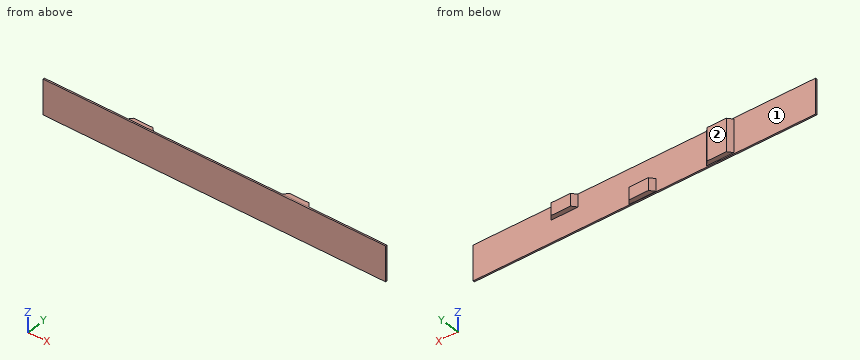
from build123d import *

# Parameters (mm, degrees)
SKETCH1_W           = 2200
SKETCH1_H           = 225
BOSS_EXTRUDE1_DEPTH = 10
BOSS_EXTRUDE2_START = 30
BOSS_EXTRUDE2_DEPTH = 80
BOSS_EXTRUDE3_START = -30
BOSS_EXTRUDE3_DEPTH = 80
BOSS_EXTRUDE4_DEPTH = 105


with BuildPart() as part:
    # Sketch1 → Boss-Extrude1 (new body)
    with BuildSketch(Plane(origin=(0, 0, 0), x_dir=(1, 0, 0), z_dir=(0, 1, 0))):
        Rectangle(SKETCH1_W, SKETCH1_H)
    extrude(amount=BOSS_EXTRUDE1_DEPTH)

    # Sketch2 → Boss-Extrude2 (add)
    with BuildSketch(Plane.XY.offset(BOSS_EXTRUDE2_START)):
        Polygon((425, 10), (450, 40), (575, 40), (600, 10), align=None)
    extrude(amount=BOSS_EXTRUDE2_DEPTH)

    # Sketch3 → Boss-Extrude3 (add)
    with BuildSketch(Plane.XY.offset(BOSS_EXTRUDE3_START)):
        Polygon((75, 40), (-50, 40), (-75, 10), (100, 10), align=None)
    extrude(amount=-BOSS_EXTRUDE3_DEPTH)

    # Sketch4 → Boss-Extrude4 (add, symmetric)
    with BuildSketch(Plane.XY):
        Polygon((-425, 40), (-550, 40), (-575, 10), (-400, 10), align=None)
    extrude(amount=BOSS_EXTRUDE4_DEPTH, both=True)


solid = part.part
The model under review builds one solid part; all positions refer to its coordinate system, in mm. Face numbers are marked on the shaded views. Coordinates: 2 decimals unless noted, no trailing zeros. Loops run counter-clockwise (first coordinate to the right, second up) from the corner with the lowest first, then second, coordinate; pieces in that order, holes last. Notation, with made-up numbers: (31.25, 26.25) -> (80.25, 26.25) arc R25 cw to (80.25, 63.25) -> close; hole circle Ø1 at (30, -17). An arc over 180 degrees is marked (long way). Use a Markdown table: item, result. Add a question column.
1. Clearance check with flat-ended pins moving along their axes: pin 1 Ø15 at (x, y) = (-20, 23.5) entering from +Z; pin 2 Ø1 at (y, z) = (16.5, -17) entering from -X; pin 3 Ø15 at (x, y) = (-482, 30.5) entering from +Z. State where each tip first meets the part, or that it passes through.
2. Add section C-C on x = 782. Write out the cut boundary in (y, z).
3. Draft analysis for pull direction X (two halves, no side actions). For the marked faces 1 and 2, state which applies: pulls with the +X half, pulls with the -X half, needs draft (parallel to the pull), parting line crosses it, or undercut.
4. Add section A-A on y = 32.5. Write out the cut boundary in (x, z), plus the area to 3 significant figures.
5. Add section B-B on z = 4. Write out the cut boundary in (x, y), plus the area to 3 significant figures.
6. To check wall thickness, follow line 1 (Y direction, x = -842.5, z = 97.5); line 2 (X direction, y = 19, z = 77); line 3 (X direction, y = 38, z = -71). State the ranges of each line that lie inside material, in increasing order.
Returned:
| question | item | result |
|---|---|---|
| 1 | pin 1 | stops at z = -30 |
| 1 | pin 2 | stops at x = -570 |
| 1 | pin 3 | stops at z = 105 |
| 2 | outline | (0, -112.5) -> (10, -112.5) -> (10, 112.5) -> (0, 112.5) -> close |
| 3 | face 1 | undercut |
| 3 | face 2 | needs draft |
| 4 | outline | (-556.25, -105) -> (-418.75, -105) -> (-418.75, 105) -> (-556.25, 105) -> close; (-56.25, -110) -> (81.25, -110) -> (81.25, -30) -> (-56.25, -30) -> close; (443.75, 30) -> (581.25, 30) -> (581.25, 110) -> (443.75, 110) -> close |
| 4 | area | 50,900 mm² |
| 5 | outline | (-1100, 0) -> (1100, 0) -> (1100, 10) -> (-400, 10) -> (-425, 40) -> (-550, 40) -> (-575, 10) -> (-1100, 10) -> close |
| 5 | area | 26,500 mm² |
| 6 | line 1 | y = 0 to 10 |
| 6 | line 2 | x = -567.5 to -407.5, 432.5 to 592.5 |
| 6 | line 3 | x = -551.67 to -423.33, -51.67 to 76.67 |
